from build123d import *

# Parameters (mm, degrees)
F0_W        = 163.068
F0_H        = 82.804
F1_DEPTH    = 9.652
F2_R        = 7.62
F3_R        = 5.08
F4_T        = -2.54
F6_W        = 8.6941672489
F6_H        = 17.6881290972
F7_DEPTH    = 25.4
F8_T1_DEPTH = 2.54


# Not quite as in the source:
# - a fillet or chamfer that OpenCascade refuses, or shapes differently, is made with other operations: its cross-section is extruded or revolved along the edge and cut away or added


with BuildPart() as f1:
    # F0 (on Top) → F1 (new body)
    with BuildSketch(Plane.XY):
        with Locations((81.534, -41.402)):
            Rectangle(F0_W, F0_H)
    extrude(amount=F1_DEPTH)

    # F2
    f2_edges = [f1.edges().sort_by_distance(p)[0] for p in [
        (0, 0, 4.826),
        (163.068, 0, 4.826),
        (163.068, -82.804, 4.826),
        (0, -82.804, 4.826),
    ]]
    fillet(f2_edges, radius=F2_R)

    # F3
    f3_edges = [f1.edges().sort_by_distance(p)[0] for p in [
        (81.534, 0, 9.652),
        (160.836154, -2.231846, 9.652),
        (2.231846, -2.231846, 9.652),
        (163.068, -41.402, 9.652),
        (0, -41.402, 9.652),
        (160.836154, -80.572154, 9.652),
        (2.231846, -80.572154, 9.652),
        (81.534, -82.804, 9.652),
    ]]
    fillet(f3_edges, radius=F3_R)

    # F4
    f4_openings = [f1.faces().sort_by_distance(p)[0] for p in [
        (81.534, -41.402, 0),
    ]]
    offset(amount=F4_T, openings=f4_openings)

    # F6 (on face) → F7 (cut)
    with BuildSketch(Plane.XY.offset(9.652)):
        with Locations((15.8525095321, -60.5635698885)):
            Rectangle(F6_W, F6_H)
    extrude(amount=-F7_DEPTH, mode=Mode.SUBTRACT)

    # F8: fillet of radius 5.08 on 4 edges, made by hand

    # F8_s2 → F8_t1 (join)
    with BuildSketch(Plane.XY.offset(7.112)):
        with BuildLine():
            ThreePointArc((11.5054259077, -56.7995053399), (12.9933234592, -53.2074028914), (16.5854259077, -51.7195053399))
            Line((16.5854259077, -51.7195053399), (11.5054259077, -51.7195053399))
            Line((11.5054259077, -51.7195053399), (11.5054259077, -56.7995053399))
        make_face()
        with BuildLine():
            ThreePointArc((11.5054259077, -64.3276344371), (12.9933234592, -67.9197368855), (16.5854259077, -69.4076344371))
            Line((16.5854259077, -69.4076344371), (11.5054259077, -69.4076344371))
            Line((11.5054259077, -69.4076344371), (11.5054259077, -64.3276344371))
        make_face()
        with BuildLine():
            ThreePointArc((20.1995931566, -56.7995053399), (18.711695605, -53.2074028914), (15.1195931566, -51.7195053399))
            Line((15.1195931566, -51.7195053399), (20.1995931566, -51.7195053399))
            Line((20.1995931566, -51.7195053399), (20.1995931566, -56.7995053399))
        make_face()
        with BuildLine():
            ThreePointArc((15.1195931566, -69.4076344371), (18.711695605, -67.9197368855), (20.1995931566, -64.3276344371))
            Line((20.1995931566, -64.3276344371), (20.1995931566, -69.4076344371))
            Line((20.1995931566, -69.4076344371), (15.1195931566, -69.4076344371))
        make_face()
    extrude(amount=F8_T1_DEPTH)


solid = f1.part
Part model, mm, in its own coordinate system. A direction names the side the tool comes from. Give positions to 0.01 mm unless a question says otherwise; leave off trailing zeros. Loops run counter-clockwise (first coordinate to the right, second up) from the corner with the lowest first, then second, coordinate; pieces in that order, holes last. Notation, with made-up numbers: M -11.5,-29.5 L 39.5,-29.5 A18 ccw 39.5,-22.5 Z; hole C 64.5,79 d10. An arc over 180 degrees is marked long. Put each result on its own line as item: value. Start each with the question number.
1) 3-axis set-ups, long thin cutter, end or side, ignore diameter. For faces 1 (the flat face through (160.528, -42, 2)), 2 (the cylindrical face through (12.71, -53.515, 8.364)), 3 (the flat face through (81, -1, 0)): which of +Z, -Z, +X, -X, +Y, -Y reach the whole face in a straight line?
2) Saw through at A-A (y = -59). List the corners of the cut face in (x, z).
3) Probe probe 1 along X at (y, z) = (-70, 3.75); probe 2 along Y at (x, z) = (52, 3.5); probe 3 along Z at (x, y) = (136.5, -53). List the from-to ranges inside material, lowest first.
4) Saw through at B-B (x = 36). List the corners of the cut face in (y, z), then the cut area to 3 significant figures.
5) Flat gauge pins, fed straight in: pin 1 (4 mm diameter, centred on x = 122, y = -58, fed in from -Z); pin 2 (3 mm diameter, centred on y = -58.5, z = 8.5, fed in from +X); pin 3 (2 mm diameter, centred on y = -62, z = 8, fed in from -X). Where does each tip first touch, or does it go through?
6) Saw through at C-C (y = -48.5). List the corners of the cut face in (x, z), then the cut area to 3 significant figures.
Numbers:
1. face 1: -Z
1. face 2: +Z, -Z
1. face 3: -Z, +X, -X, +Y, -Y
2. outline: M 0,0 L 2.54,0 L 2.54,4.57 A2.54 cw 5.08,7.11 L 11.51,7.11 L 11.51,9.65 L 5.08,9.65 A5.08 ccw 0,4.57 Z; M 20.2,7.11 L 157.99,7.11 A2.54 cw 160.53,4.57 L 160.53,0 L 163.07,0 L 163.07,4.57 A5.08 ccw 157.99,9.65 L 20.2,9.65 Z
3. probe 1: 0 to 2.54, 160.53 to 163.07
3. probe 2: -82.8 to -80.26, -2.54 to 0
3. probe 3: 7.11 to 9.65
4. outline: M -82.8,0 L -80.26,0 L -80.26,4.57 A2.54 cw -77.72,7.11 L -5.08,7.11 A2.54 cw -2.54,4.57 L -2.54,0 L 0,0 L 0,4.57 A5.08 ccw -5.08,9.65 L -77.72,9.65 A5.08 ccw -82.8,4.57 Z
4. area: 238 mm^2
5. pin 1: z = 7.11
5. pin 2: x = 162.45
5. pin 3: x = 0.62
6. outline: M 0,0 L 2.54,0 L 2.54,4.57 A2.54 cw 5.08,7.11 L 157.99,7.11 A2.54 cw 160.53,4.57 L 160.53,0 L 163.07,0 L 163.07,4.57 A5.08 ccw 157.99,9.65 L 5.08,9.65 A5.08 ccw 0,4.57 Z
6. area: 442 mm^2
